```python
from build123d import *

# Parameters (mm, degrees)
SKETCH1_W           = 185
SKETCH1_H           = 185
SKETCH1_R           = 1.5
BOSS_EXTRUDE1_DEPTH = 2
CUT_EXTRUDE1_DEPTH  = 2
FILLET1_R           = 10
SKETCH3_R           = 2.5
CUT_EXTRUDE2_DEPTH  = 262.637153325


with BuildPart() as part:
    # Sketch1 → Boss-Extrude1 (new body)
    with BuildSketch(Plane(origin=(0, 0, 0), x_dir=(1, 0, 0), z_dir=(0, 1, 0))):
        with Locations((92.5, 92.5)):
            Rectangle(SKETCH1_W, SKETCH1_H)
        with Locations(Location((86.843145751, 98.156854249, 0), (0, 0, 270))):
            Circle(SKETCH1_R, mode=Mode.SUBTRACT)
        with Locations(Location((98.156854249, 98.156854249, 0), (0, 0, 270))):
            Circle(SKETCH1_R, mode=Mode.SUBTRACT)
        with Locations(Location((98.156854249, 86.843145751, 0), (0, 0, 270))):
            Circle(SKETCH1_R, mode=Mode.SUBTRACT)
        with Locations(Location((86.843145751, 86.843145751, 0), (0, 0, 270))):
            Circle(SKETCH1_R, mode=Mode.SUBTRACT)
    extrude(amount=BOSS_EXTRUDE1_DEPTH)

    # Sketch2 → Cut-Extrude1 (cut)
    with BuildSketch(Plane(origin=(0, 2, 0), x_dir=(1, 0, 0), z_dir=(0, 1, 0))):
        with BuildLine():
            ThreePointArc((18, 177), (16.141462703, 176.825774225), (14.347686426, 176.309167823))
            Line((14.347686426, 176.309167823), (92.5, 98.156854249))
            Line((92.5, 98.156854249), (170.652313574, 176.309167823))
            ThreePointArc((170.652313574, 176.309167823), (168.858537297, 176.825774225), (167, 177))
            Line((167, 177), (18, 177))
        make_face()
        with BuildLine():
            Line((86.843145751, 92.5), (8.690832177, 170.652313574))
            ThreePointArc((8.690832177, 170.652313574), (8.174225583, 168.858536282), (8, 166.999997934))
            Line((8, 166.999997934), (8, 18))
            ThreePointArc((8, 18), (8.174225775, 16.141462703), (8.690832177, 14.347686426))
            Line((8.690832177, 14.347686426), (86.843145751, 92.5))
        make_face()
        with BuildLine():
            Line((170.652313574, 8.690832177), (92.5, 86.843145751))
            Line((92.5, 86.843145751), (14.347686426, 8.690832177))
            ThreePointArc((14.347686426, 8.690832177), (16.141462703, 8.174225775), (18, 8))
            Line((18, 8), (167, 8))
            ThreePointArc((167, 8), (168.858537297, 8.174225775), (170.652313574, 8.690832177))
        make_face()
        with BuildLine():
            Line((176.309167823, 170.652313574), (98.156854249, 92.5))
            Line((98.156854249, 92.5), (176.309167823, 14.347686426))
            ThreePointArc((176.309167823, 14.347686426), (176.825774033, 16.141461688), (177, 17.999997934))
            Line((177, 17.999997934), (177, 167))
            ThreePointArc((177, 167), (176.825774225, 168.858537297), (176.309167823, 170.652313574))
        make_face()
    extrude(amount=-CUT_EXTRUDE1_DEPTH, mode=Mode.SUBTRACT)

    # Fillet1
    fillet1_edges = [part.edges().sort_by_distance(p)[0] for p in [
        (0, 1, -185),
        (185, 1, -185),
        (185, 1, 0),
        (0, 1, 0),
    ]]
    fillet(fillet1_edges, radius=FILLET1_R)

    # Sketch3 → Cut-Extrude2 (cut, through all)
    with BuildSketch(Plane(origin=(0, 2, 0), x_dir=(1, 0, 0), z_dir=(0, 1, 0))):
        with Locations(Location((7.878679656, 177.121320344, 0), (0, 0, 270))):
            Circle(SKETCH3_R)
        with Locations(Location((177.121320344, 177.121320344, 0), (0, 0, 270))):
            Circle(SKETCH3_R)
        with Locations(Location((177.121320344, 7.878679656, 0), (0, 0, 270))):
            Circle(SKETCH3_R)
        with Locations(Location((7.878679656, 7.878679656, 0), (0, 0, 270))):
            Circle(SKETCH3_R)
    extrude(amount=-CUT_EXTRUDE2_DEPTH, mode=Mode.SUBTRACT)


solid = part.part
```
Read the model definition and answer for the solid it produces. Units are mm, in the model's axes. A direction names the side the tool comes from. Give positions to 0.01 mm unless a question says otherwise; leave off trailing zeros. Write each loop counter-clockwise with the first axis right and the second up, starting at its lowest first coordinate (ties: lowest second). Pieces come first, ordered by that corner, then holes. Notation, with made-up numbers: (50, 86) - (60, 86) arc R18 ccw to (60, 119) - close; hole circle Ø2 at (42, 20.5). An arc over 180 degrees is marked (long way). Write item = value, one per line. Start each with the question number.
Item 1: Find section A-A (z = -40.5). Give the vertices of the cut face in (x, y).
Item 2: Find section C-C (y = 1.2). State how many separate pieces and enclosed holes the cut face has, then the cut area to 3 significant figures.
Item 3: The mould has two halves that part along Z. Classify faces 1 (the cylindrical face through (181.99, 1.01, -182.15)), 2 (the flat face through (137.78, 1.014, -132.123)), 3 (the flat face through (136.686, 1.014, -53.971)), 4 (the cylindrical face through (181.99, 1.01, -2.85)): +Z half, -Z half, draft (parallel to the pull), parting line (faces both ways), or undercut.
Item 4: Find the intervals of material crossed by probe 1 along Z at (x, y) = (16.5, 0.4); probe 2 along Z at (x, y) = (167, 0.75); probe 3 along X at (y, z) = (0.2, -66), in increasing order. Write a range as [from, to].
Item 5: A tool of negligible diameter and unlimited length cuts with its end or side. For faces 5 (the cylindrical face through (2.85, 1.01, -3.01)), 6 (the flat face through (53.971, 1.014, -48.314)), from which of +Z, -Z, +X, -X, +Y, -Y can it reach the whole face along a straight path? Write none if from no direction.
Item 6: Find section B-B (x = 64.5). Give the vertices of the cut face in (y, z).
Response:
q1.outline = (0, 0) - (8, 0) - (8, 2) - (0, 2) - close; (34.84, 0) - (46.16, 0) - (46.16, 2) - (34.84, 2) - close; (138.84, 0) - (150.16, 0) - (150.16, 2) - (138.84, 2) - close; (177, 0) - (185, 0) - (185, 2) - (177, 2) - close
q2.separate_pieces = 1
q2.enclosed_holes = 12
q2.area = 9,180 mm²
q3.face_1 = -Z half
q3.face_2 = undercut
q3.face_3 = undercut
q3.face_4 = +Z half
q4.probe_1 = [-185, -176.89], [-174.16, -162.84], [-22.16, -10.84], [-8.11, 0]
q4.probe_2 = [-185, -177], [-172.66, -161.34], [-23.66, -12.34], [-8, 0]
q4.probe_3 = [0, 8], [60.34, 71.66], [113.34, 124.66], [177, 185]
q5.face_5 = +Z, -X, +Y, -Y
q5.face_6 = +Y, -Y
q6.outline = (0, -185) - (2, -185) - (2, -177) - (0, -177) - close; (0, -126.16) - (2, -126.16) - (2, -114.84) - (0, -114.84) - close; (0, -70.16) - (2, -70.16) - (2, -58.84) - (0, -58.84) - close; (0, -8) - (2, -8) - (2, 0) - (0, 0) - close
